Build history of the part. All positions in model axes, mm. Face numbers are marked on the shaded views. A direction names the side the tool comes from. Round coordinates to 2 decimals unless told otherwise and drop trailing zeros. Write each loop counter-clockwise with the first axis right and the second up, starting at its lowest first coordinate (ties: lowest second). Pieces come first, ordered by that corner, then holes.
Item 1: Drop flat-ended pins along their axis: pin 1 Ø5 at (y, z) = (62.5, -18) entering from -X; pin 2 Ø9 at (x, y) = (5, 22) entering from +Z; pin 3 Ø5 at (x, y) = (30, 40) entering from -Z. Give the stop position or say it passes through.
Item 2: Band-saw the part on B-B, the plane y = 40. Write the cut outline in (x, z).
Item 3: Band-saw the part on D-D, the plane y = 22. Write the cut outline in (x, z), then the cut area to 3 significant figures.
Item 4: 3-axis set-ups, long thin cutter, end or side, ignore diameter. For the marked faces 1 and 2: which of +Z, -Z, +X, -X, +Y, -Y reach the whole face in a straight line?
Item 5: Wall check: probe 1 along Y at (x, z) = (55, -9.25); probe 2 along Y at (x, z) = (5, -17.5); probe 3 along X at (y, z) = (53.5, -3). Give the ranges that are in metal, low to high.
Item 6: Band-saw the part on C-C, the plane z = -5.5. Write the cut outline in (x, y), then the cut area to 3 significant figures.
Item 7: Band-saw the part on A-A, the plane x = 5. Write the cut outline in (y, z).
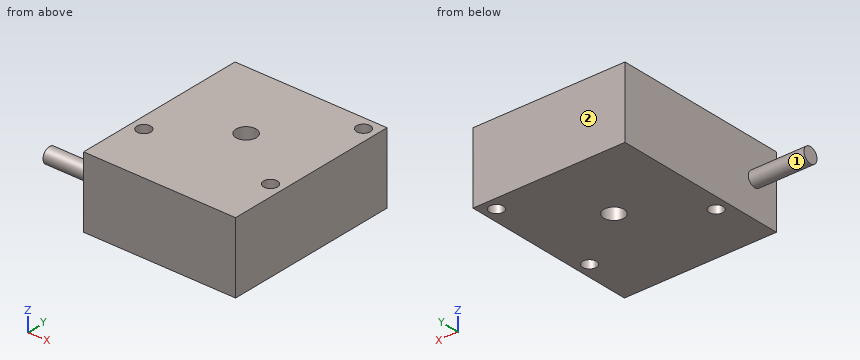
```python
from build123d import *

# Parameters (mm, degrees)
ESQUISSE1_W      = 60
ESQUISSE1_H      = 70
EXTRUSION1_DEPTH = 28
ESQUISSE2_R      = 3
EXTRUSION2_DEPTH = 22
EXTRUSION3_REACH = 98.354
ESQUISSE3_R      = 4
D_GAGEMENT_M51_D = 5.5


with BuildPart() as part:
    # Esquisse1 → Extrusion1 (new body)
    with BuildSketch(Plane.XY):
        with Locations((30, 35)):
            Rectangle(ESQUISSE1_W, ESQUISSE1_H)
    extrude(amount=-EXTRUSION1_DEPTH)

    # Esquisse2 → Extrusion2 (add)
    with BuildSketch(Plane.ZY):
        with Locations((-14, 10)):
            Circle(ESQUISSE2_R)
    extrude(amount=EXTRUSION2_DEPTH)

    # Esquisse3 → Extrusion3 (cut, up to next)
    with BuildSketch(Plane.XY, mode=Mode.PRIVATE) as extrusion3_sk1:
        with Locations((30, 40)):
            Circle(ESQUISSE3_R)
    extrusion3_tool1 = extrude(extrusion3_sk1.sketch, amount=-EXTRUSION3_REACH, mode=Mode.PRIVATE) & part.part
    add(extrusion3_tool1.solids().sort_by_distance((30, 40, 0))[0], mode=Mode.SUBTRACT)

    # Dégagement M51 (through all)
    with Locations(Plane(origin=(55, 22, -28), x_dir=(-1, 0, 0), z_dir=(0, 0, -1))):
        with Locations((0, 0), (0, 43), (50, 0)):
            Hole(D_GAGEMENT_M51_D / 2)


solid = part.part
```
Results:
1. pin 1: stops at x = 0
1. pin 2: stops at z = 0
1. pin 3: passes through
2. outline: (0, -28) - (26, -28) - (26, 0) - (0, 0) - close; (34, -28) - (60, -28) - (60, 0) - (34, 0) - close
3. outline: (0, -28) - (2.25, -28) - (2.25, 0) - (0, 0) - close; (7.75, -28) - (52.25, -28) - (52.25, 0) - (7.75, 0) - close; (57.75, -28) - (60, -28) - (60, 0) - (57.75, 0) - close
3. area: 1,370 mm2
4. face 1: -X
4. face 2: +Z, -Z, +X, -X, +Y
5. probe 1: y = 0 to 19.25, 24.75 to 62.25, 67.75 to 70
5. probe 2: y = 0 to 19.25, 24.75 to 70
5. probe 3: x = 0 to 60
6. outline: (0, 0) - (60, 0) - (60, 70) - (0, 70) - close; hole circle Ø5.5 at (5, 22); hole circle Ø8 at (30, 40); hole circle Ø5.5 at (55, 22); hole circle Ø5.5 at (55, 65)
6. area: 4,080 mm2
7. outline: (0, -28) - (19.25, -28) - (19.25, 0) - (0, 0) - close; (24.75, -28) - (70, -28) - (70, 0) - (24.75, 0) - close
